Could you check a few things on this model? Use its own coordinates, in mm. A direction names the side the tool comes from. Round coordinates to 2 decimals unless told otherwise and drop trailing zeros. Write each loop counter-clockwise with the first axis right and the second up, starting at its lowest first coordinate (ties: lowest second). Pieces come first, ordered by that corner, then holes. Notation, with made-up numbers: (9.25, -25) -> (57.25, -25) arc R15 ccw to (57.25, -21) -> close; hole circle Ø1 at (65, -23.5). An arc over 180 degrees is marked (long way). One line per question, with ' | ' between items. Start each with the question number.
1. Imagine slicing it at C-C, the plane z = 19. List the corners of the cut face in (x, y) for me.
2. If I drill on line 1 along X through (y, z) = (-30, 13.5); line 2 along Y through (x, z) = (-5.75, 14.5); line 3 along Z through (x, y) = (-9.5, -32), over which ranges is the centre line in solid material (lowest first)? Write a range as [from, to].
3. For faces 1 (the flat face through (-5.046, -14, 9)), 2 (the flat face through (-15, -18, 4.83)), which set-ups out of +Z, -Z, +X, -X, +Y, -Y let a thin tool reach every point of the face, with its end or its side?
4. Thinking about a two-plate mould opening in Z: for faces 3 (the cylindrical face through (-14.91, -18.91, -6.82)), 4 (the flat face through (-15, -5.798, 16)), 5 (the cylindrical face through (-8.99, -13.53, 14.67)), which applies, released by +Z, released by -Z, zero draft, split by the parting line, or undercut?
5. Imagine slicing it at A-A, the plane y = -15. List the corners of the cut face in (x, z) for me, and give its area (3 significant figures).
6. Imagine slicing it at D-D, the plane z = 10.5. List the corners of the cut face in (x, y) for me, and give its area (3 significant figures).
7. Imagine slicing it at B-B, the plane x = -13.5. List the corners of the cut face in (y, z) for me, and give its area (3 significant figures).
8. For pin 1 Ø3 at (y, z) = (-16, 12) entering from -X; pin 2 Ø2 at (x, z) = (-17.5, 3) entering from -Y; pin 3 Ø3 at (x, y) = (-21.5, -34) entering from -Z; pin 4 Ø5 at (x, y) = (-11.5, -5.5) entering from -Z, each with a flat end and sliding along its axis, tell me the tip position at first contact or that it passes through.
from build123d import *

# Parameters (mm, degrees)
BOSS_EXTRU_1_START      = -10
BOSS_EXTRU_1_DEPTH      = 80
ESQUISSE3_W             = 16
ESQUISSE3_H             = 100
ENL_V_MAT_EXTRU_1_DEPTH = 80
BOSS_EXTRU_2_DEPTH      = 80
CONG_1_R                = 11
ENL_V_MAT_EXTRU_2_REACH = 146.791
ESQUISSE8_R             = 20
ESQUISSE9_R             = 5
ENL_V_MAT_EXTRU_3_DEPTH = 80
ECHELLE1_SCALE          = 0.25


with BuildPart() as part:
    # Esquisse2 → Boss.-Extru.1 (new body)
    with BuildSketch(Plane.XY.offset(BOSS_EXTRU_1_START)):
        Polygon((-55.04572219, 21.601620468), (-55.04572219, -49.548379532), (-55.04572219, -83.308379532), (24.95427781, -83.308379532), (24.95427781, -43.249651956), (24.95427781, 27.900348044), (24.95427781, 46.691620468), (-55.04572219, 46.691620468), align=None)
    extrude(amount=BOSS_EXTRU_1_DEPTH)

    # Esquisse3 → Enlèv. mat.-Extru.1 (cut)
    with BuildSketch(Plane.XY.offset(70)):
        with Locations((-15.04572219, -18.308379532)):
            Rectangle(ESQUISSE3_W, ESQUISSE3_H)
    extrude(amount=-ENL_V_MAT_EXTRU_1_DEPTH, mode=Mode.SUBTRACT)

    # Esquisse6 → Boss.-Extru.2 (add)
    with BuildSketch(Plane(origin=(24.95427781, 0, 0), x_dir=(0, 0, -1), z_dir=(1, 0, 0))):
        with BuildLine():
            Line((-70, 46.691620468), (10, 46.691620468))
            Line((10, 46.691620468), (10, -83.308379532))
            Line((10, -83.308379532), (-70, -83.308379532))
            ThreePointArc((-70, -83.308379532), (56.636895265, -18.308379532), (-70, 46.691620468))
        make_face()
    extrude(amount=-BOSS_EXTRU_2_DEPTH)

    # Congé1
    cong_1_edges = [part.edges().sort_by_distance(p)[0] for p in [
        (-15.04572219, 31.691620468, -10),
        (-15.04572219, -68.308379532, -10),
    ]]
    fillet(cong_1_edges, radius=CONG_1_R)

    # Enlèv. mat.-Extru.2: up to this face of the body (flat: up to its plane)
    enl_v_mat_extru_2_end = Plane(part.part.faces().sort_by_distance((-55.04572219, -18.308379532, 12.636185619))[0])
    # Esquisse8 → Enlèv. mat.-Extru.2 (cut, up to the picked face)
    with BuildSketch(Plane(origin=(24.95427781, 0, 0), x_dir=(0, 0, -1), z_dir=(1, 0, 0)), mode=Mode.PRIVATE) as enl_v_mat_extru_2_sk1:
        with Locations(Location((-23.363104735, -18.308379532, 0), (0, 0, 90))):
            Circle(ESQUISSE8_R)
    enl_v_mat_extru_2_tool1 = split(extrude(enl_v_mat_extru_2_sk1.sketch, amount=-ENL_V_MAT_EXTRU_2_REACH, mode=Mode.PRIVATE), bisect_by=enl_v_mat_extru_2_end, keep=Keep.BOTH, mode=Mode.PRIVATE)
    add(enl_v_mat_extru_2_tool1.solids().sort_by(Axis((24.954278, -18.30838, 23.363105), (-1, 0, 0)))[0], mode=Mode.SUBTRACT)

    # Esquisse9 → Enlèv. mat.-Extru.3 (cut)
    with BuildSketch(Plane.ZY.offset(55.04572219)):
        with Locations(Location((26.681094555, 37.25802852, 0), (0, 0, 270))):
            Circle(ESQUISSE9_R)
        with Locations(Location((26.681094555, -76.2999152, 0), (0, 0, 270))):
            Circle(ESQUISSE9_R)
    extrude(amount=-ENL_V_MAT_EXTRU_3_DEPTH, mode=Mode.SUBTRACT)


with BuildPart() as part_1:
    # Echelle1: scaled about (-15.04572219, -18.295074577, 9.77346256)
    add(part.part.scale(ECHELLE1_SCALE).moved(Location((-11.284291642, -13.721305933, 7.33009692))))


solid = part_1.part
Geometry results:
1) outline: (-25.05, -37.43) -> (-5.05, -37.43) -> (-5.05, 0.83) -> (-25.05, 0.83) -> close; hole (-17.05, -30.8) -> (-13.05, -30.8) -> (-13.05, -5.8) -> (-17.05, -5.8) -> close
2) line 1: x = [-25.05, -17.05], [-13.05, -5.05] | line 2: y = [-38.25, -33.94], [-31.65, -23.12], [-13.48, -5.55], [-3.26, 1.66] | line 3: z = [-1.4, 13.04], [14.96, 24.83]
3) face 1: +Z, -Z, +X, +Y, -Y | face 2: +Z
4) face 3: split by the parting line | face 4: zero draft | face 5: undercut
5) outline: (-25.05, -6.56) -> (-5.05, -6.56) -> (-5.05, 9.41) -> (-13.05, 9.41) -> (-13.05, 4.83) -> (-17.05, 4.83) -> (-17.05, 9.41) -> (-25.05, 9.41) -> close; (-25.05, 16.93) -> (-17.05, 16.93) -> (-17.05, 24.83) -> (-25.05, 24.83) -> close; (-13.05, 16.93) -> (-5.05, 16.93) -> (-5.05, 24.83) -> (-13.05, 24.83) -> close | area: 427 mm2
6) outline: (-25.05, -38.12) -> (-5.05, -38.12) -> (-5.05, -22.53) -> (-13.05, -22.53) -> (-13.05, -30.8) -> (-17.05, -30.8) -> (-17.05, -22.53) -> (-25.05, -22.53) -> close; (-25.05, -14.07) -> (-17.05, -14.07) -> (-17.05, -5.8) -> (-13.05, -5.8) -> (-13.05, -14.07) -> (-5.05, -14.07) -> (-5.05, 1.52) -> (-25.05, 1.52) -> close | area: 558 mm2
7) outline: (-34.55, 24.83) arc R20 ccw (long way) to (-2.05, 24.83) -> (-5.8, 24.83) -> (-5.8, 7.58) arc R2.75 cw to (-8.55, 4.83) -> (-28.05, 4.83) arc R2.75 cw to (-30.8, 7.58) -> (-30.8, 24.83) -> close; hole circle Ø2.5 at (-32.8, 14); hole circle Ø2.5 at (-4.41, 14) | area: 560 mm2
8) pin 1: passes through | pin 2: stops at y = -36.07 | pin 3: stops at z = -0.91 | pin 4: stops at z = -3.97
